Read the model definition and answer for the solid it produces. Units are mm, in the model's axes. Coordinates: 2 decimals unless noted, no trailing zeros. Write each loop counter-clockwise with the first axis right and the second up, starting at its lowest first coordinate (ties: lowest second). Pieces come first, ordered by that corner, then holes. Notation, with made-up numbers: (67, 46) - (78, 46) arc R11 ccw to (78, 51) - close; hole circle Ø5 at (-10.5, 51.25). An arc over 180 degrees is marked (long way). Return JSON: item names as keys, results as strings.
Autodesk Inventor part; units mm, degrees
ref_plane "YZ Plane" through (0, 0, 0) normal (1, 0, 0) x (0, 1, 0)
ref_plane "XZ Plane" through (0, 0, 0) normal (0, 1, 0) x (-1, 0, 0)
ref_plane "XY Plane" through (0, 0, 0) normal (0, 0, 1) x (1, 0, 0)
sketch "Sketch1" plane through (0, 0, 0) normal (1, 0, 0) x (0, 1, 0)
  line L0 (0, 0) -> (50.8, 0)
  line L1 (50.8, 0) -> (50.8, -25.4)
  line L2 (50.8, -25.4) -> (0, -25.4)
  line L3 (0, -25.4) -> (0, 0)
  line L4 (2.54, -2.54) -> (48.26, -2.54)
  line L5 (48.26, -2.54) -> (48.26, -22.86)
  line L6 (48.26, -22.86) -> (2.54, -22.86)
  line L7 (2.54, -22.86) -> (2.54, -2.54)
  dimension "d0" = 50.8
  dimension "d1" = 25.4
  dimension "d2" = 45.72
  dimension "d3" = 20.32
  dimension "d4" = 2.54
  dimension "d5" = 2.54
extrude "Extrusion1" add sketch "Sketch1" along normal blind 711.2
sketch "Sketch2" plane through (0, 50.8, 0) normal (0, 1, 0) x (1, 0, 0)
  line L0 (0, 0) -> (0, 25.4)
  line L1 (0, 0) -> (711.2, 0)
  line L2 (711.2, 25.4) -> (711.2, 0)
  line L3 (0, 25.4) -> (711.2, 25.4)
  line L4 (0, 2.54) -> (0, 22.86)
  point P0 (12.7, 12.7)
  dimension "d9" = 12.7
  dimension "d10" = 12.7
hole "Hole1" at (12.7, 50.8, -12.7) direction (0, -1, 0) diameter 3.9688 end through all
pattern_linear "Rectangular Pattern1" count 28 spacing 25.4 along (1, 0, 0) of "Hole1"
sketch "Sketch6" plane through (0, 50.8, 0) normal (0, 1, 0) x (1, 0, 0)
  circle A0 centre (698.5, 12.7) radius 1.9844
  circle A1 centre (673.1, 12.7) radius 1.9844
  circle A2 centre (647.7, 12.7) radius 1.9844
  circle A3 centre (622.3, 12.7) radius 1.9844
  circle A4 centre (596.9, 12.7) radius 1.9844
  circle A5 centre (571.5, 12.7) radius 1.9844
  circle A6 centre (546.1, 12.7) radius 1.9844
  circle A7 centre (520.7, 12.7) radius 1.9844
  circle A8 centre (495.3, 12.7) radius 1.9844
  circle A9 centre (469.9, 12.7) radius 1.9844
  circle A10 centre (444.5, 12.7) radius 1.9844
  circle A11 centre (419.1, 12.7) radius 1.9844
  circle A12 centre (393.7, 12.7) radius 1.9844
  circle A13 centre (368.3, 12.7) radius 1.9844
  circle A14 centre (342.9, 12.7) radius 1.9844
  circle A15 centre (317.5, 12.7) radius 1.9844
  circle A16 centre (292.1, 12.7) radius 1.9844
  circle A17 centre (266.7, 12.7) radius 1.9844
  circle A18 centre (241.3, 12.7) radius 1.9844
  circle A19 centre (215.9, 12.7) radius 1.9844
  circle A20 centre (190.5, 12.7) radius 1.9844
  circle A21 centre (165.1, 12.7) radius 1.9844
  circle A22 centre (139.7, 12.7) radius 1.9844
  circle A23 centre (114.3, 12.7) radius 1.9844
  circle A24 centre (88.9, 12.7) radius 1.9844
  circle A25 centre (63.5, 12.7) radius 1.9844
  circle A26 centre (38.1, 12.7) radius 1.9844
  circle A27 centre (12.7, 12.7) radius 1.9844
  line L0 (0, 0) -> (0, 25.4)
  line L1 (0, 0) -> (711.2, 0)
  line L2 (711.2, 25.4) -> (711.2, 0)
  line L3 (0, 25.4) -> (711.2, 25.4)
  circle A28 centre (139.7, 12.7) radius 1.9844
  circle A29 centre (139.7, 12.7) radius 3.175
  circle A30 centre (266.7, 12.7) radius 3.175
  circle A31 centre (571.5, 12.7) radius 3.175
  circle A32 centre (444.5, 12.7) radius 1.9844
  circle A33 centre (444.5, 12.7) radius 3.175
  circle A34 centre (698.5, 12.7) radius 1.9844
  circle A35 centre (698.5, 12.7) radius 3.175
  circle A36 centre (12.7, 12.7) radius 3.175
  dimension "d58" = 6.35
  dimension "d59" = 6.35
  dimension "d60" = 6.35
  dimension "d61" = 6.35
  dimension "d62" = 6.35
  dimension "d63" = 6.35
extrude "Extrusion4" cut sketch "Sketch6" against normal blind 50.8 contours A29 | A30 | A31 | A33 | A35 | A36
sketch "Sketch7" plane through (0, 50.8, 0) normal (0, 1, 0) x (1, 0, 0)
  line L0 (0, 25.4) -> (711.2, 25.4)
  circle A0 centre (698.5, 12.7) radius 3.175
  circle A1 centre (571.5, 12.7) radius 3.175
  circle A2 centre (139.7, 12.7) radius 3.175
  circle A3 centre (266.7, 12.7) radius 3.175
  circle A4 centre (444.5, 12.7) radius 3.175
  circle A5 centre (12.7, 12.7) radius 3.175
  circle A6 centre (673.1, 12.7) radius 1.9844
  circle A7 centre (647.7, 12.7) radius 1.9844
  circle A8 centre (622.3, 12.7) radius 1.9844
  circle A9 centre (596.9, 12.7) radius 1.9844
  circle A10 centre (546.1, 12.7) radius 1.9844
  circle A11 centre (520.7, 12.7) radius 1.9844
  circle A12 centre (495.3, 12.7) radius 1.9844
  circle A13 centre (469.9, 12.7) radius 1.9844
  circle A14 centre (419.1, 12.7) radius 1.9844
  circle A15 centre (393.7, 12.7) radius 1.9844
  circle A16 centre (368.3, 12.7) radius 1.9844
  circle A17 centre (342.9, 12.7) radius 1.9844
  circle A18 centre (317.5, 12.7) radius 1.9844
  circle A19 centre (292.1, 12.7) radius 1.9844
  circle A20 centre (241.3, 12.7) radius 1.9844
  circle A21 centre (215.9, 12.7) radius 1.9844
  circle A22 centre (190.5, 12.7) radius 1.9844
  circle A23 centre (165.1, 12.7) radius 1.9844
  circle A24 centre (114.3, 12.7) radius 1.9844
  circle A25 centre (88.9, 12.7) radius 1.9844
  circle A26 centre (63.5, 12.7) radius 1.9844
  circle A27 centre (38.1, 12.7) radius 1.9844
  line L1 (0, 0) -> (0, 25.4)
  line L2 (0, 0) -> (711.2, 0)
  line L3 (711.2, 25.4) -> (711.2, 0)
  line L4 (0, 25.4) -> (711.2, 25.4)
  point P0 (127, 12.7)
  point P1 (101.6, 12.7)
  point P2 (76.2, 12.7)
  point P3 (50.8, 12.7)
  point P4 (584.2, 12.7)
  point P5 (609.6, 12.7)
  point P6 (635, 12.7)
  point P7 (660.4, 12.7)
  dimension "d66" = 12.7
  dimension "d67" = 12.7
  dimension "d68" = 12.7
  dimension "d69" = 12.7
  dimension "d70" = 50.8
  dimension "d71" = 76.2
  dimension "d72" = 101.6
  dimension "d73" = 127
  dimension "d74" = 50.8
  dimension "d75" = 76.2
  dimension "d76" = 101.6
  dimension "d77" = 127
  dimension "d78" = 12.7
  dimension "d79" = 12.7
  dimension "d80" = 12.7
  dimension "d81" = 12.7
hole "Hole3" at (127, 50.8, -12.7) at (101.6, 50.8, -12.7) at (76.2, 50.8, -12.7) at (50.8, 50.8, -12.7) at (584.2, 50.8, -12.7) at (609.6, 50.8, -12.7) at (635, 50.8, -12.7) at (660.4, 50.8, -12.7) direction (0, -1, 0) diameter 3.9688 end through all
properties part number "frame_wide"
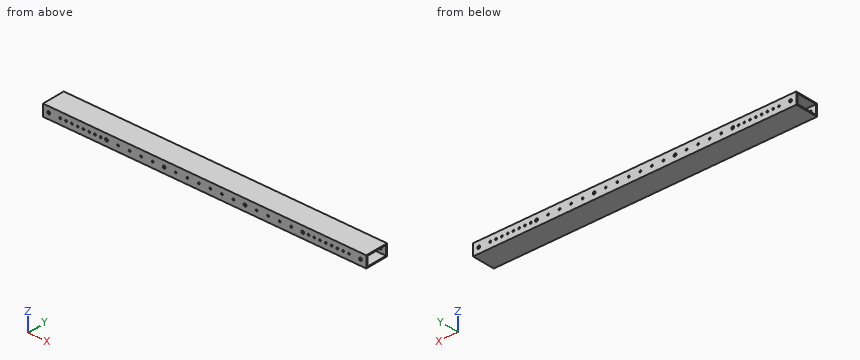
(1) Straight lines are drawn through the part: line 1 (Y direction, x = 116.5, z = -4.5); line 2 (Z direction, x = 561, y = 13); line 3 (Z direction, x = 596.9, y = 48.85). For each, find the intervals that lie inside material, in ascending order. Write a range as from..to.
Answer:
{"line 1": "0..2.54, 48.26..50.8", "line 2": "-25.4..-22.86, -2.54..0", "line 3": "-25.4..-14.68, -10.72..0"}
(2) Flat-ended cylindrical pins translate along their axes: P1, Ø3, axis at x = 78.5, z = -18.5, coming from the -Y side; P2, Ø2.5, axis at x = 419.1, z = -12.7, coming from the -Y side. Find the tip coordinate at first contact, or state that the pin passes through.
Answer:
{"P1": "y = 0", "P2": "through"}
(3) A cutting plane is placed at A-A (y = 17.5). Determine the outline of the cut face in (x, z), and give its area (3 significant figures).
Answer:
{"outline": "(0, -25.4) - (711.2, -25.4) - (711.2, -22.86) - (0, -22.86) - close; (0, -2.54) - (711.2, -2.54) - (711.2, 0) - (0, 0) - close", "area": "3,610 mm²"}
